Design review of the part built by this model. Coordinates are the model's own, in mm. A direction names the side the tool comes from. Coordinates: 2 decimals unless noted, no trailing zeros. Order: outer loops, then holes, each group sorted by start corner. A loop starts at its lowest first (then second) coordinate and runs counter-clockwise, first axis right, second up.
Autodesk Inventor part; units mm, degrees
ref_plane "YZ Plane" through (0, 0, 0) normal (1, 0, 0) x (0, 1, 0)
ref_plane "XZ Plane" through (0, 0, 0) normal (0, 1, 0) x (-1, 0, 0)
ref_plane "XY Plane" through (0, 0, 0) normal (0, 0, 1) x (1, 0, 0)
ref_plane "Płaszczyzna konstrukcyjna1" through (0, 0, 0) normal (0, 0, 1) x (1, 0, 0)
sketch "Szkic1" plane through (0, 0, 0) normal (0, 0, 1) x (1, 0, 0)
  circle A0 centre (0, 0) radius 72.5
  circle A1 centre (0, 0) radius 35.3971
  arc A2 (19.3649, 5) -> (19.3649, -5) centre (0, 0) ccw
  line L0 (24, 5) -> (24, -5)
  line L1 (24, -5) -> (19.3649, -5)
  line L2 (19.3649, 5) -> (24, 5)
extrude "Wyciągnięcie proste1" add sketch "Szkic1" along normal blind 25 contours A0 | A1
sketch "Szkic2" plane through (0, 0, 25) normal (0, 0, 1) x (1, 0, 0)
  circle A0 centre (62.5, 0) radius 2.4585
  point P0 (0, 0)
hole "Otwór1" at (62.5, 0, 25) direction (0, 0, -1) diameter 5 end through all
pattern_circular "Szyk kołowy1" count 6 over 360 about axis through (0, 0, -10) along (0, 0, 1) of "Otwór1"
properties material "Stal nierdzewna"
1. Mouldability with a two-part tool opening along Y and no side actions: class faces 1 (the flat face through (15, -15, 0)), 2 (the cylindrical face through (69.15, -21.78, 12.32)), 3 (the cylindrical face through (-64.72, 1.15, 12.32)) as pulls with the +Y half, pulls with the -Y half, needs draft (parallel to the pull), parting line crosses it, or undercut.
2. To check wall thickness, follow line 1 (Y direction, x = -33, z = 11.5); line 2 (Y direction, x = -31.5, z = 23.5); line 3 (Y direction, x = 7, z = 12.5). State the ranges of each line that lie inside material, in increasing order.
3. Add section C-C (x = 31.25). Give the boundary of the cut face in (y, z), and give its area (3 significant figures).
4. Add section B-B (y = 10). Give the boundary of the cut face in (x, z).
5. Add section A-A (x = 0). Give the boundary of the cut face in (y, z), and give its area (4 significant figures).
6. Add section D-D (z = 4.75). Give the boundary of the cut face in (x, y), and give its area (3 significant figures).
7. For faces 4 (the flat face through (24, 0, 12)), 5 (the flat face through (15, -15, 25)), list the 3-axis set-ups (+Z, -Z, +X, -X, +Y, -Y) from which the entire face can be reached by the end or side of a thin tool; tool diameter is ignored.
8. Insertion check: pin 1 (12 mm diameter, centred on y = -4, z = 16.5, fed in from -X); pin 2 (2 mm diameter, centred on y = 17, z = 11.5, fed in from +X); pin 3 (4 mm diameter, centred on x = -7, z = 13, fed in from -Y); pin 4 (5 mm diameter, centred on y = 48.5, z = 14, fed in from +X). Each pin has a flat end and moves straight along its axis. Give the tip position at first contact, or say it passes through.
Solution:
1. face 1: needs draft
1. face 2: parting line crosses it
1. face 3: undercut
2. line 1: y = -64.55 to -55.91, -52.34 to 52.34, 55.91 to 64.55
2. line 2: y = -65.3 to -56.61, -51.64 to 51.64, 56.61 to 65.3
2. line 3: y = -72.16 to -18.73, 18.73 to 72.16
3. outline: (-65.42, 0) - (-56.63, 0) - (-56.63, 25) - (-65.42, 25) - close; (-51.63, 0) - (51.63, 0) - (51.63, 25) - (-51.63, 25) - close; (56.63, 0) - (65.42, 0) - (65.42, 25) - (56.63, 25) - close
3. area: 3,020 mm2
4. outline: (-71.81, 0) - (-17.32, 0) - (-17.32, 25) - (-71.81, 25) - close; (17.32, 0) - (71.81, 0) - (71.81, 25) - (17.32, 25) - close
5. outline: (-72.5, 0) - (-20, 0) - (-20, 25) - (-72.5, 25) - close; (20, 0) - (72.5, 0) - (72.5, 25) - (20, 25) - close
5. area: 2,625 mm2
6. outline: circle Ø145 at (0, 0); hole circle Ø5 at (-62.5, 0); hole circle Ø5 at (-31.25, -54.13); hole circle Ø5 at (-31.25, 54.13); hole (19.36, -5) - (24, -5) - (24, 5) - (19.36, 5) arc R20 ccw (long way) to start; hole circle Ø5 at (31.25, -54.13); hole circle Ø5 at (31.25, 54.13); hole circle Ø5 at (62.5, 0)
6. area: 15,100 mm2
7. face 4: +Z, -Z
7. face 5: +Z, +X, -X, +Y, -Y
8. pin 1: stops at x = -72.5
8. pin 2: stops at x = 70.71
8. pin 3: stops at y = -72.33
8. pin 4: stops at x = 56.04
